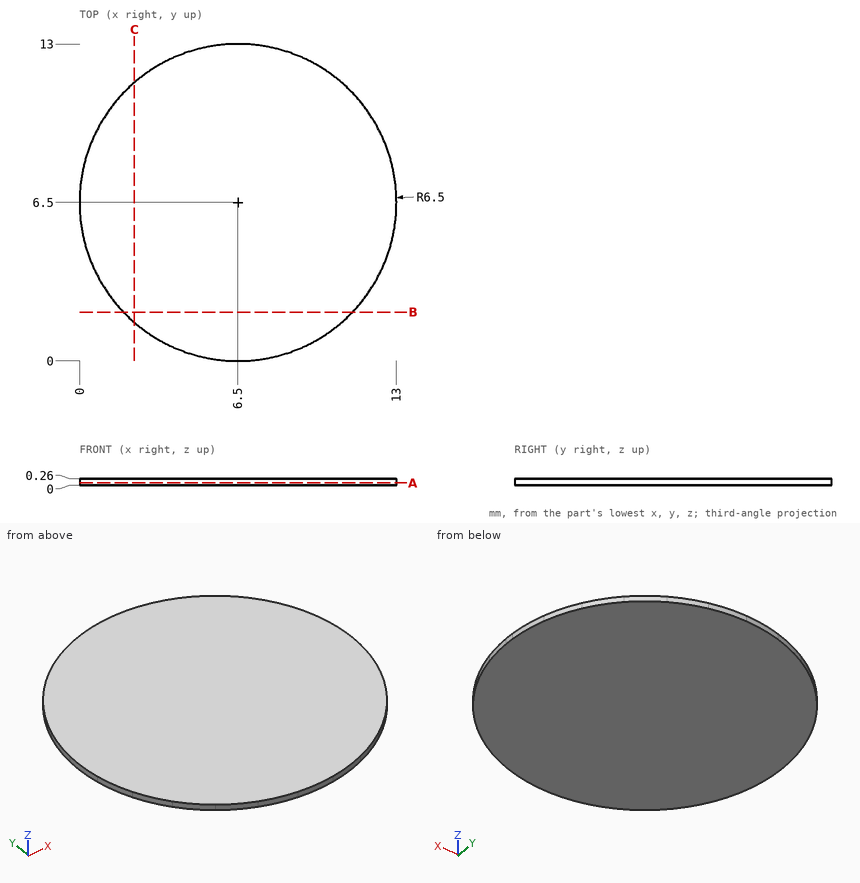
Drawing for the job (mm, zero at the part's lowest x, y, z). Coordinates: 2 decimals unless noted, no trailing zeros. Order: outer loops, then holes, each group sorted by start corner. A loop starts at its lowest first (then second) coordinate and runs counter-clockwise, first axis right, second up. Notation, with made-up numbers: (35.5, -34.5) -> (39.5, -34.5) arc R23 cw to (39.5, 0.5) -> close; hole circle Ø6 at (85, 27.5). An arc over 180 degrees is marked (long way). Answer in a Markdown table with one row per item.
1) Drill centre lines: line 1 (X direction, y = 4.5, z = 0.05); line 2 (X direction, y = 3.5, z = 0.15); line 3 (Y direction, x = 11, z = 0.15). Where is each one in solid material? Low to high.
Check values:
| item | result |
|---|---|
| line 1 | 0.32 to 12.68 |
| line 2 | 0.73 to 12.27 |
| line 3 | 1.81 to 11.19 |
2) Band-saw the part on A-A (z = 0.1). List the corners of the cut face in (x, y), and give its area (3 significant figures).
Check values:
| item | result |
|---|---|
| outline | circle Ø13 at (6.5, 6.5) |
| area | 133 mm2 |
3) Flat gauge pin, fed straight in: P1, Ø1, axis at x = 2, y = 7, coming from the -Z side. Where does the tip first touch, or does it go through?
Check values:
| item | result |
|---|---|
| P1 | z = 0 |
4) Band-saw the part on C-C (x = 2.25). List the corners of the cut face in (y, z).
Check values:
| item | result |
|---|---|
| outline | (1.58, 0) -> (11.42, 0) -> (11.42, 0.26) -> (1.58, 0.26) -> close |
5) Band-saw the part on B-B (y = 2). List the corners of the cut face in (x, z).
Check values:
| item | result |
|---|---|
| outline | (1.81, 0) -> (11.19, 0) -> (11.19, 0.26) -> (1.81, 0.26) -> close |
